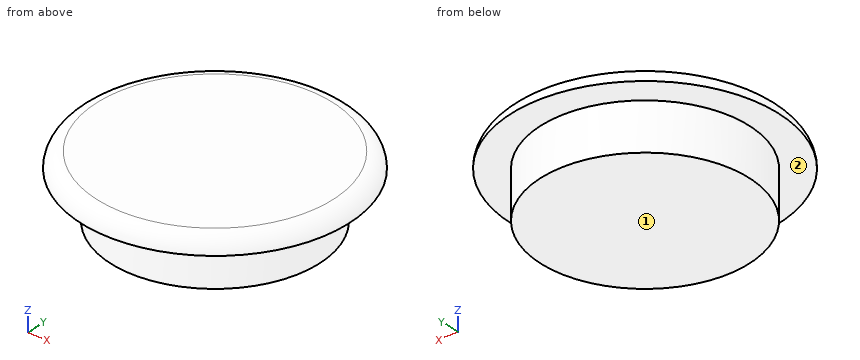
Autodesk Fusion 360 part; units mm, degrees
sketch "Skizze1" plane through (0, 0, 0) normal (0, 0, 1) x (1, 0, 0)
  circle A0 centre (0, 0) radius 13.25
  dimension "d1" = 26.5
extrude "Extrusion1" add sketch "Skizze1" along normal blind 6
sketch "Skizze2" plane through (0, 0, 6) normal (0, 0, 1) x (-1, 0, 0)
  circle A0 centre (0, 0) radius 13.25
  circle A1 centre (0, 0) radius 17
  dimension "d4" = 34
extrude "Extrusion2" add sketch "Skizze2" along normal blind 2 contours A0 | A1
fillet "Abrundung1" radius 2 1 edges at (15.8496, 6.1475, 8)
CAD build for the part. Positions are in the model's coordinates, mm. Face numbers are marked on the shaded views. A direction names the side the tool comes from. Coordinates: 2 decimals unless noted, no trailing zeros. Write each loop counter-clockwise with the first axis right and the second up, starting at its lowest first coordinate (ties: lowest second). Pieces come first, ordered by that corner, then holes. Notation, with made-up numbers: M -29.5,11.25 L -12.5,11.25 A16 ccw -12.5,29.25 Z; hole C -34,86.5 d9. An arc over 180 degrees is marked long. Return JSON: item names as keys, results as strings.
Item 1: Probe line 1 (Z direction, x = 4, y = 14); line 2 (Y direction, x = -8, z = 1.25); line 3 (X direction, y = -0.5, z = 7.5). List the from-to ranges inside material, lowest first. Write a range as from..to.
Findings below:
{"line 1": "z = 6..8", "line 2": "y = -10.56..10.56", "line 3": "x = -16.32..16.32"}
Item 2: Slice it at C-C, the plane z = 5.5. Write the cut outline in (x, y).
Findings below:
{"outline": "C 0,0 d26.5"}
Item 3: Drop a flat-ended pin along its axis: pin 1 Ø1.5 at (y, z) = (3.5, 6) entering from -X. Give the stop position or say it passes through.
Findings below:
{"pin 1": "stops at x = -16.78"}
Item 4: Which spindle directions (+Z, -Z, +X, -X, +Y, -Y) get a long thin tool onto all of the face, cutting with end or side? Do the marked faces 1 and 2. Say none if no direction does.
Findings below:
{"face 1": "-Z, +X, -X, +Y, -Y", "face 2": "-Z"}
